```python
from build123d import *

# Parameters (mm, degrees)
F1_W     = 30
F1_H     = 32.3
F2_DEPTH = 5.5
F0_W     = 12.5
F0_H     = 22.9
F3_DEPTH = 7
F4_W     = 8.75
F4_H     = 4.9
F4_W_2   = 12.5
F4_H_2   = 22.9
F4_H_3   = 4.5
F5_DEPTH = 20
F6_SIZE  = 2
F7_SIZE  = 2


with BuildPart() as f2:
    # F1 (on Top) → F2 (new body)
    with BuildSketch(Plane.XY):
        with Locations((6.25, 11.25)):
            Rectangle(F1_W, F1_H)
    extrude(amount=F2_DEPTH)

    # F0 (on Top) → F3 (cut)
    with BuildSketch(Plane.XY):
        with Locations((6.25, 11.45)):
            Rectangle(F0_W, F0_H)
    extrude(amount=F3_DEPTH, mode=Mode.SUBTRACT)

    # F4 (on Top) → F5 (join)
    with BuildSketch(Plane.XY):
        with Locations((-4.375, -2.45)):
            Rectangle(F4_W, F4_H)
        with Locations((6.25, -2.45)):
            Rectangle(F4_W_2, F4_H)
        with Locations((-4.375, 11.45)):
            Rectangle(F4_W, F4_H_2)
        with Locations((-4.375, 25.15)):
            Rectangle(F4_W, F4_H_3)
        with Locations((16.875, 11.45)):
            Rectangle(F4_W, F4_H_2)
        with Locations((16.875, -2.45)):
            Rectangle(F4_W, F4_H)
        with Locations((16.875, 25.15)):
            Rectangle(F4_W, F4_H_3)
    extrude(amount=-F5_DEPTH)

    # F6
    f6_edges = [f2.edges().sort_by_distance(p)[0] for p in [
        (6.25, 0, 5.5),
    ]]
    chamfer(f6_edges, length=F6_SIZE)

    # F7
    f7_edges = [f2.edges().sort_by_distance(p)[0] for p in [
        (6.25, 0, 3.5),
    ]]
    chamfer(f7_edges, length=F7_SIZE)


solid = f2.part
```
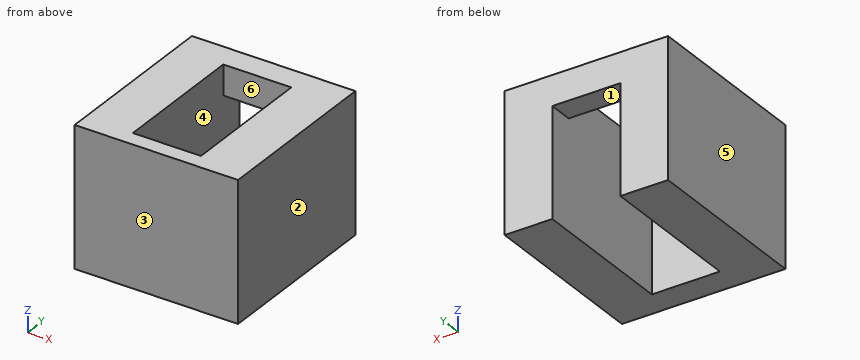
Check sheet for the modelled part. Datum: model origin and axes. Units: mm. Face numbers are marked on the shaded views. A direction names the side the tool comes from. Round coordinates to 2 decimals unless told otherwise and drop trailing zeros. Loops run counter-clockwise (first coordinate to the right, second up) from the corner with the lowest first, then second, coordinate; pieces in that order, holes last. Notation, with made-up numbers: (5, 71) - (61, 71) arc R17 cw to (61, 100) - close; hole circle Ø1 at (48.25, 22). An arc over 180 degrees is marked (long way). Write item = value, one per line. Start each with the question number.
Q1. Depth check by flat-ended pin: P1, Ø6, axis at x = 5, z = -5, coming from the +Y side; P2, Ø2, axis at x = 8, y = 1.5, coming from the +Z side; P3, Ø1.3, axis at x = 8.5, y = 25, coming from the -Z side. Enter the tip coordinate at first touch or a pass-through.
Q2. Access from +Z, -Z, +X, -X, +Y, -Y to the whole of each face (thin tool, end or side, straight path). Record for the marked faces 1 and 2.
Q3. Section check A-A (y = 22). Record the boundary of the cut face in (x, z).
Q4. Thickness scan on L1, parallel to X at y = 25.5, z = -14.75; L2, parallel to Z at x = 9.5, y = 24; L3, parallel to Y at x = 3, z = -6.75. Record the ranges inside material, lowest first.
Q5. Section check D-D (z = 0.5). Record the boundary of the cut face in (x, y), plus the area to 3 significant figures.
Q6. Section check C-C (z = -8.5). Record the boundary of the cut face in (x, y).
Q7. Section check B-B (x = 2.25). Record the boundary of the cut face in (y, z).
Q8. Release check for a two-part mould opening along X. For the marked faces 3, 4, 5 and 6 record: pulls with the +X half, pulls with the -X half, needs draft (parallel to the pull), parting line crosses it, or undercut.
Derived:
q1.P1 = 0
q1.P2 = through
q1.P3 = 0
q2.face_1 = -Z, +Y
q2.face_2 = +Z, -Z, +X, +Y, -Y
q3.outline = (-8.75, -20) - (0, -20) - (0, 5.5) - (-8.75, 5.5) - close; (12.5, -20) - (21.25, -20) - (21.25, 5.5) - (12.5, 5.5) - close
q4.L1 = -8.75 to 0, 12.5 to 21.25
q4.L2 = 0 to 5.5
q4.L3 = -4.9 to 0
q5.outline = (-8.75, -4.9) - (21.25, -4.9) - (21.25, 27.4) - (-8.75, 27.4) - close; hole (0, 0) - (12.5, 0) - (12.5, 22.9) - (0, 22.9) - close
q5.area = 683 mm^2
q6.outline = (-8.75, -4.9) - (21.25, -4.9) - (21.25, 27.4) - (12.5, 27.4) - (12.5, 0) - (0, 0) - (0, 27.4) - (-8.75, 27.4) - close
q7.outline = (-4.9, -20) - (0, -20) - (0, 1.5) - (-1.41, 4.91) - (-2, 5.5) - (-4.9, 5.5) - close; (22.9, 0) - (27.4, 0) - (27.4, 5.5) - (22.9, 5.5) - close
q8.face_3 = needs draft
q8.face_4 = undercut
q8.face_5 = pulls with the -X half
q8.face_6 = undercut
